The listing builds one solid part. Answer for the finished solid, in the listing's coordinates (mm). A direction names the side the tool comes from. Give positions to 0.01 mm unless a question says otherwise; leave off trailing zeros. Order: outer loops, then holes, each group sorted by start corner. A loop starts at its lowest first (then second) coordinate and runs counter-clockwise, first axis right, second up. Notation, with made-up numbers: (-19.5, 41.5) - (5.5, 41.5) arc R26 cw to (5.5, 71.5) - close; hole circle Ø6 at (3.25, 58.25). An arc over 180 degrees is marked (long way). Use CSV: the item, a comma, the result in double quotes.
```python
from build123d import *

# Parameters (mm, degrees)
FILLET_R     = 0.2
POCKET_DEPTH = 0.5
FILLET001_R  = 0.05


with BuildPart() as part:
    # Sketch → Revolution (revolve)
    with BuildSketch(Plane.XY):
        Polygon((0, 0), (0, 8.3), (1.55, 8.3), (1.55, 7), (1, 7), (1, 0), align=None)
    revolve(axis=Axis((0, 0, 0), (0, 1, 0)))

    # Fillet
    fillet_edges = [part.edges().sort_by_distance(p)[0] for p in [
        (-1.55, 8.3, 0),
        (-1.55, 7, 0),
    ]]
    fillet(fillet_edges, radius=FILLET_R)

    # Sketch001 (on Face1 of Fillet) → Pocket (cut)
    with BuildSketch(Plane(origin=(0, 8.3, 0), x_dir=(-1, 0, 0), z_dir=(0, 1, 0))):
        Polygon((0, 1), (0.3, 1), (0.3, 0.3), (1, 0.3), (1, -0.3), (0.3, -0.3), (0.3, -1), (0, -1), align=None)
    pocket = extrude(amount=-POCKET_DEPTH, mode=Mode.SUBTRACT)

    # Mirrored: Pocket across Sketch001 V_Axis
    add(pocket.mirror(Plane(origin=(0, 8.3, 0), x_dir=(0, 1, 0), z_dir=(-1, 0, 0))), mode=Mode.SUBTRACT)

    # Fillet001
    fillet001_edges = [part.edges().sort_by_distance(p)[0] for p in [
        (-0.65, 8.3, 0.3),
        (-1, 8.3, 0),
        (-0.65, 8.3, -0.3),
        (-0.3, 8.3, -0.65),
        (-0.15, 8.3, -1),
        (0.15, 8.3, -1),
        (0.3, 8.3, -0.65),
        (0.65, 8.3, -0.3),
        (0.65, 8.3, 0.3),
        (1, 8.3, 0),
        (0.3, 8.3, 0.65),
        (-0.3, 8.3, 0.65),
        (-0.15, 8.3, 1),
        (0.15, 8.3, 1),
    ]]
    fillet(fillet001_edges, radius=FILLET001_R)


solid = part.part
```
Item 1: Which of the six approach directions +Z, -Z, +X, -X, +Y, -Y give full straight-line access (tool end or side, diameter ignored) to faces 4 (the face through (-0.6, 8.3, 0.6)), 5 (the face through (0, 3, 1))?
Taken from the geometry:
face 4,"+Z, -Z, +X, -X, +Y"
face 5,"-Y"
Item 2: The mould has two halves that part along X. Classify faces 1 (the face through (0.715, 7.644, 1.375)), 2 (the face through (0, 7.8, 0)), 3 (the face through (0, 0, 0)): +X half, -X half, draft (parallel to the pull), parting line (faces both ways), or undercut.
Taken from the geometry:
face 1,"parting line"
face 2,"undercut"
face 3,"draft"
Item 3: The part is cut by section C-C (y = 1.75). Give the vertices of the cut face in (x, z).
Taken from the geometry:
outline,"circle Ø2 at (0, 0)"
Item 4: Find the intervals of material crossed by line 1 along Y through (x, z) = (0.4, 1.1); line 2 along Z through (x, y) = (0.05, 6.5); line 3 along Y through (x, z) = (0.55, 0.2), in increasing order.
Taken from the geometry:
line 1,"7 to 8.3"
line 2,"-1 to 1"
line 3,"0 to 7.8"
Item 5: The part is cut by section A-A (z = 0). Give the vertices of the cut face in (x, y), and give its area (3 significant figures).
Taken from the geometry:
outline,"(-1.55, 7.2) arc R0.2 ccw to (-1.35, 7) - (-1, 7) - (-1, 0) - (1, 0) - (1, 7) - (1.35, 7) arc R0.2 ccw to (1.55, 7.2) - (1.55, 8.1) arc R0.2 ccw to (1.35, 8.3) - (1.05, 8.3) arc R0.05 ccw to (1, 8.25) - (1, 7.8) - (-1, 7.8) - (-1, 8.25) arc R0.05 ccw to (-1.05, 8.3) - (-1.35, 8.3) arc R0.2 ccw to (-1.55, 8.1) - close"
area,"17.0 mm^2"
Item 6: Each of these flat-tipped pins is pushed along its axis until it touches: pin 1 (1 mm diameter, centred on y = 3, z = -1, fed in from -X); pin 2 (1 mm diameter, centred on y = 2, z = 0.5, fed in from -X); pin 3 (0.8 mm diameter, centred on x = -0.5, z = 0.5, fed in from -Y); pin 4 (1 mm diameter, centred on x = 1, y = 2.5, fed in from -Z). Where does it stop, or does it pass through?
Taken from the geometry:
pin 1,"x = -0.87"
pin 2,"x = -1"
pin 3,"y = 0"
pin 4,"z = -0.87"
Item 7: The part is cut by section B-B (x = 0). Give the vertices of the cut face in (y, z).
Taken from the geometry:
outline,"(0, -1) - (7, -1) - (7, -1.35) arc R0.2 ccw to (7.2, -1.55) - (8.1, -1.55) arc R0.2 ccw to (8.3, -1.35) - (8.3, -1.05) arc R0.05 ccw to (8.25, -1) - (7.8, -1) - (7.8, 1) - (8.25, 1) arc R0.05 ccw to (8.3, 1.05) - (8.3, 1.35) arc R0.2 ccw to (8.1, 1.55) - (7.2, 1.55) arc R0.2 ccw to (7, 1.35) - (7, 1) - (0, 1) - close"
